Check sheet for the modelled part. Datum: model origin and axes. Units: mm. A direction names the side the tool comes from. Give positions to 0.01 mm unless a question says otherwise; leave off trailing zeros. Order: outer loops, then holes, each group sorted by start corner. A loop starts at its lowest first (then second) coordinate and runs counter-clockwise, first axis right, second up. Notation, with made-up numbers: (3.5, -8.5) - (55.5, -8.5) arc R19 ccw to (55.5, 7.5) - close; hole circle Ø9 at (28.25, -20). An arc over 180 degrees is marked (long way). Answer in a Markdown table with one row per item.
Autodesk Inventor part; units mm, degrees
ref_plane "YZ Plane" through (0, 0, 0) normal (1, 0, 0) x (0, 1, 0)
ref_plane "XZ Plane" through (0, 0, 0) normal (0, 1, 0) x (-1, 0, 0)
ref_plane "XY Plane" through (0, 0, 0) normal (0, 0, 1) x (1, 0, 0)
sketch "Sketch1" plane through (0, 0, 0) normal (0, 1, 0) x (-1, 0, 0)
  line L0 (0, 0) -> (40, 0)
  line L1 (40, 0) -> (40, -20)
  line L2 (40, -20) -> (0, -20)
  line L3 (0, -20) -> (0, 0)
  dimension "d0" = 40
  dimension "d1" = 20
extrude "Extrusion1" add sketch "Sketch1" along normal blind 4
sketch "Sketch2" plane through (0, 4, 0) normal (0, 1, 0) x (1, 0, 0)
  circle A0 centre (-30, 10) radius 2.75
  circle A1 centre (-10, 10) radius 2.75
  line L0 (0, 20) -> (-40, 20)
  line L1 (-40, 20) -> (-40, 0)
  point P0 (0, 0)
  dimension "d4" = 5.5
  dimension "d5" = 5.5
  dimension "d6" = 10
  dimension "d7" = 10
  dimension "d8" = 20
extrude "Extrusion2" cut sketch "Sketch2" against normal through all
sketch "Sketch3" plane through (0, 4, 0) normal (0, 1, 0) x (1, 0, 0)
  line L0 (-40, 20) -> (-40, 0)
  line L1 (-40, 0) -> (0, 0)
  line L2 (0, 0) -> (0, 4)
  line L3 (0, 4) -> (-40, 4)
  line L4 (-40, 4) -> (-40, 0)
  dimension "d11" = 40
  dimension "d12" = 4
extrude "Extrusion3" add sketch "Sketch3" along normal blind 36
sketch "Sketch4" plane through (0, 4, -4) normal (0, 0, -1) x (-1, 0, 0)
  circle A0 centre (10, 26) radius 2.75
  line L0 (0, 0) -> (0, 36)
  line L1 (0, 36) -> (40, 36)
  point P0 (0, -4)
  dimension "d15" = 5.5
  dimension "d16" = 10
  dimension "d17" = 10
extrude "Extrusion4" cut sketch "Sketch4" against normal through all
pattern_linear "Rectangular Pattern1" count 2 spacing 20 along (0, -1, 0) count 2 spacing 20 along (-1, 0, 0) of "Extrusion4"
sketch "Sketch5" plane through (0, 0, 0) normal (1, 0, 0) x (0, 0, -1)
  line L0 (4, 4) -> (4, 40)
  line L1 (20, 4) -> (4, 4)
  line L2 (4, 40) -> (20, 4)
  line L3 (20, 4) -> (4, 4)
  line L4 (4, 4) -> (4, 40)
  point P0 (0, 0)
extrude "Extrusion5" add sketch "Sketch5" against normal blind 3
pattern_linear "Rectangular Pattern2" count 2 spacing 37 along (-1, 0, 0) of "Extrusion5"
fillet "Fillet1" radius 2 4 edges at (-20, 4, -20) (-20, 40, -4) (-3, 22, -12) (-37, 22, -12)
properties part number "Bottom_Bracket"
(1) Cross-section at B-B, the plane x = -6. Record the cut outline in (y, z), then the cut area to 3 significant figures.
Geometry says:
| item | result |
|---|---|
| outline | (0, -20) - (2, -20) arc R2 ccw to (4, -18) - (4, -4) - (38, -4) arc R2 ccw to (40, -2) - (40, 0) - (0, 0) - close |
| area | 222 mm² |
(2) Cross-section at A-A, the plane x = -10. Record the cut outline in (y, z), then the cut area to 3 significant figures.
Geometry says:
| item | result |
|---|---|
| outline | (0, -20) - (2, -20) arc R2 ccw to (4, -18) - (4, -12.75) - (0, -12.75) - close; (0, -7.25) - (4, -7.25) - (4, -4) - (7.25, -4) - (7.25, 0) - (0, 0) - close; (12.75, -4) - (27.25, -4) - (27.25, 0) - (12.75, 0) - close; (32.75, -4) - (38, -4) arc R2 ccw to (40, -2) - (40, 0) - (32.75, 0) - close |
| area | 156 mm² |
(3) Gauge pin test, flat ends, axial feed: P1, Ø11, axis at x = -16, z = -10, coming from the +Y side; P2, Ø3, axis at x = -33, y = 22.5, coming from the -Z side; P3, Ø1, axis at x = -33.5, z = -4, coming from the +Y side. Record the tip position at first contact, or that the pin passes through.
Geometry says:
| item | result |
|---|---|
| P1 | y = 4 |
| P2 | z = -4 |
| P3 | y = 39.32 |
(4) Access from +Z, -Z, +X, -X, +Y, -Y to the whole of each face (thin tool, end or side, straight path). Record for faces 4 (the flat face through (-20, 21, -4)), 5 (the cylindrical face through (-8.52, 2.03, -12.32)).
Geometry says:
| item | result |
|---|---|
| face 4 | -Z, +Y |
| face 5 | +Y, -Y |
(5) Thickness scan on L1, parallel to X at y = 1.4, z = -10; L2, parallel to Y at x = -30, z = -1.45; L3, parallel to Z at x = -10, y = 1. Record the ranges inside material, lowest first.
Geometry says:
| item | result |
|---|---|
| L1 | -40 to -32.75, -27.25 to -12.75, -7.25 to 0 |
| L2 | 0 to 7.25, 12.75 to 27.25, 32.75 to 40 |
| L3 | -20 to -12.75, -7.25 to 0 |
(6) Mould release check, pull along Y, two halves, no side actions. Record for faces 1 (the cylindrical face through (-37.6, 21.04, -11.8)), 2 (the cylindrical face through (-11.48, 12.32, -2.03)), 3 (the flat face through (-37, 13, -8)): pulls with the +Y half, pulls with the -Y half, needs draft (parallel to the pull), parting line crosses it, or undercut.
Geometry says:
| item | result |
|---|---|
| face 1 | pulls with the +Y half |
| face 2 | undercut |
| face 3 | needs draft |
(7) Cross-section at C-C, the plane z = -12. Give the number of separate pieces and of enclosed holes in the cut face, then the cut area to 3 significant figures.
Geometry says:
| item | result |
|---|---|
| separate pieces | 3 |
| enclosed holes | 0 |
| area | 234 mm² |
